Here's how the part is built. I have some questions about the finished solid (model axes, mm). A direction names the side the tool comes from. Round coordinates to 2 decimals unless told otherwise and drop trailing zeros. Loops run counter-clockwise (first coordinate to the right, second up) from the corner with the lowest first, then second, coordinate; pieces in that order, holes last. Notation, with made-up numbers: M 57.5,-10.75 L 68.5,-10.75 A18 ccw 68.5,-2.75 Z; hole C 6.25,-36 d2. An arc over 180 degrees is marked long. Use a Markdown table: item, result.
```python
from build123d import *

# Parameters (mm, degrees)
EXTRUDE_1_DEPTH          = 200
SKETCH_2_W               = 39
SKETCH_2_H               = 25
CUT_EXTRUDE_1_DEPTH      = 20
SKETCH_3_W               = 126
SKETCH_3_H               = 160
CUT_EXTRUDE_2_DEPTH      = 180
CUT_EXTRUDE_3_REACH      = 362.633
SKETCH_4_R               = 51
SKETCH_5_R               = 25.5
CUT_EXTRUDE_4_DEPTH      = 15
SKETCH_6_R               = 57.15
CUT_EXTRUDE_5_DEPTH      = 5
PATTERN_CIRCULAR_1_COUNT = 4


with BuildPart() as part:
    # 草图1 → 凸台-拉伸1 (new body)
    with BuildSketch(Plane.XY):
        Polygon((20, 225), (20, 250), (0, 250), (0, 0), (20, 0), (20, 25), (166, 25), (166, 225), align=None)
    extrude(amount=-EXTRUDE_1_DEPTH)

    # 草图2 → 切除-拉伸1 (cut)
    with BuildSketch(Plane.ZY):
        with Locations((-180.5, 237.5)):
            Rectangle(SKETCH_2_W, SKETCH_2_H)
        with Locations((-180.5, 12.5)):
            Rectangle(SKETCH_2_W, SKETCH_2_H)
    extrude(amount=-CUT_EXTRUDE_1_DEPTH, mode=Mode.SUBTRACT)

    # 草图3 → 切除-拉伸2 (cut)
    with BuildSketch(Plane(origin=(0, 0, -200), x_dir=(-1, 0, 0), z_dir=(0, 0, -1))):
        with Locations((-83, 122.583335177)):
            Rectangle(SKETCH_3_W, SKETCH_3_H)
    extrude(amount=-CUT_EXTRUDE_2_DEPTH, mode=Mode.SUBTRACT)

    # 草图4 → 切除-拉伸3 (cut, up to next)
    with BuildSketch(Plane(origin=(166, 0, 0), x_dir=(0, 0, -1), z_dir=(1, 0, 0)), mode=Mode.PRIVATE) as cut_extrude_3_sk1:
        with Locations((100, 125)):
            Circle(SKETCH_4_R)
    cut_extrude_3_tool1 = extrude(cut_extrude_3_sk1.sketch, amount=-CUT_EXTRUDE_3_REACH, mode=Mode.PRIVATE) & part.part
    add(cut_extrude_3_tool1.solids().sort_by_distance((166, 125, -100))[0], mode=Mode.SUBTRACT)

    # 草图5 → 切除-拉伸4 (cut)
    with BuildSketch(Plane(origin=(20, 0, 0), x_dir=(0, 0, -1), z_dir=(1, 0, 0))):
        with Locations(Location((100, 125, 0), (0, 0, 90))):
            Circle(SKETCH_5_R)
    extrude(amount=-CUT_EXTRUDE_4_DEPTH, mode=Mode.SUBTRACT)

    # 草图6 → 切除-拉伸5 (cut)
    with BuildSketch(Plane.ZY):
        with Locations((-100, 125)):
            Circle(SKETCH_6_R)
    extrude(amount=-CUT_EXTRUDE_5_DEPTH, mode=Mode.SUBTRACT)

    # 草图9 → M12 螺纹孔1 (revolve, cut)
    with BuildSketch(Plane(origin=(166, 195.711356231, -170.71), x_dir=(0, 0, -1), z_dir=(0, 1, 0))):
        Polygon((0, 0), (0, 29.25), (5.1, 26.185610843), (5.1, 0), align=None)
    hole_wizard_m12_1 = revolve(axis=Axis((172.35, 195.711356231, -170.71), (-1, 0, 0)), mode=Mode.SUBTRACT)

    # 阵列(圆周)1: M12 螺纹孔1 ×4 about axis
    pattern_circular_1_axis = Axis((0, 125, -100), (1, 0, 0))
    for i in range(1, PATTERN_CIRCULAR_1_COUNT):
        add(hole_wizard_m12_1.rotate(pattern_circular_1_axis, i * 360 / PATTERN_CIRCULAR_1_COUNT), mode=Mode.SUBTRACT)


solid = part.part
```
Q1. For faces 4 (the flat face through (5, 100, -88)), 5 (the flat face through (20, 12, -79)), 6 (the cylindrical face through (156.14, 57.735, -33.049)), 7 (the flat face through (84, 42.583, -111)), 8 (the flat face through (20, 237, -79)), which set-ups out of +Z, -Z, +X, -X, +Y, -Y let a thin tool reach every point of the face, with its end or its side?
Return value:
| item | result |
|---|---|
| face 4 | -X |
| face 5 | +Z, -Z, +X, -Y |
| face 6 | +X |
| face 7 | -Z |
| face 8 | +Z, -Z, +X, +Y |
Q2. I need wall thicknesses on line 1 (Y direction, x = 156, z = -29.29); line 2 (Y direction, x = 104, z = -31); line 3 (Z direction, x = 14, y = 125). Which ranges of each line are inside material? Lowest first, please. Write a range as from..to.
Return value:
| item | result |
|---|---|
| line 1 | y = 25..49.19, 59.39..190.61, 200.81..225 |
| line 2 | y = 25..42.58, 202.58..225 |
| line 3 | z = -200..-125.5, -74.5..0 |
Q3. Imagine slicing it at D-D, the plane z = -65. Please give me the cut outline in (x, y).
Return value:
| item | result |
|---|---|
| outline | M 0,0 L 20,0 L 20,25 L 166,25 L 166,87.91 L 146,87.91 L 146,42.58 L 20,42.58 L 20,202.58 L 146,202.58 L 146,162.09 L 166,162.09 L 166,225 L 20,225 L 20,250 L 0,250 L 0,170.18 L 5,170.18 L 5,79.82 L 0,79.82 Z |
Q4. We'd pull the mould along Y, two halves only. Please class faces 1 (the flat face through (8, 126, -200)), 2 (the cylindrical face through (156.14, 105.467, -147.111)), 3 (the flat face through (10, 250, -79)): pulls with the +Y half, pulls with the -Y half, needs draft (parallel to the pull), parting line crosses it, or undercut.
Return value:
| item | result |
|---|---|
| face 1 | needs draft |
| face 2 | undercut |
| face 3 | pulls with the +Y half |
Q5. Will these pins go through, and if not, where does the flat tip stop? P1, Ø9, axis at y = 195.71, z = -170.71, coming from the +X side; P2, Ø6, axis at y = 187.5, z = -24, coming from the -X side; P3, Ø5, axis at x = 72, z = -116, coming from the +Y side; P4, Ø8, axis at x = 68, y = 121.5, coming from the -Z side.
Return value:
| item | result |
|---|---|
| P1 | stops at x = 20 |
| P2 | stops at x = 0 |
| P3 | stops at y = 225 |
| P4 | stops at z = -20 |
Q6. Imagine slicing it at C-C, the plane x = 26. Please give me the cut outline in (y, z).
Return value:
| item | result |
|---|---|
| outline | M 25,-200 L 42.58,-200 L 42.58,-20 L 202.58,-20 L 202.58,-200 L 225,-200 L 225,0 L 25,0 Z |
Q7. Imagine slicing it at B-B, the plane z = -100. Please give me the cut outline in (x, y), then the cut area to 3 significant figures.
Return value:
| item | result |
|---|---|
| outline | M 0,0 L 20,0 L 20,25 L 166,25 L 166,74 L 146,74 L 146,42.58 L 20,42.58 L 20,99.5 L 5,99.5 L 5,67.85 L 0,67.85 Z; M 0,182.15 L 5,182.15 L 5,150.5 L 20,150.5 L 20,202.58 L 146,202.58 L 146,176 L 166,176 L 166,225 L 20,225 L 20,250 L 0,250 Z |
| area | 10,700 mm^2 |
Q8. Imagine slicing it at A-A, the plane y = 125. Please give me the cut outline in (x, z), then the cut area to 3 significant figures.
Return value:
| item | result |
|---|---|
| outline | M 0,-200 L 20,-200 L 20,-125.5 L 5,-125.5 L 5,-157.15 L 0,-157.15 Z; M 0,-42.85 L 5,-42.85 L 5,-74.5 L 20,-74.5 L 20,-20 L 146,-20 L 146,-49 L 166,-49 L 166,0 L 0,0 Z; M 146,-200 L 166,-200 L 166,-151 L 146,-151 Z |
| area | 7,140 mm^2 |
